```python
from build123d import *

# Parameters (mm, degrees)
SKETCH1_W                = 180
SKETCH1_H                = 110
BOSS_EXTRUDE1_DEPTH      = 50
BOSS_EXTRUDE2_DEPTH      = 110
CUT_EXTRUDE1_DEPTH       = 146.344418537
BOSS_EXTRUDE5_DEPTH      = 10
BOSS_EXTRUDE5_DEPTH_BACK = 10
SKETCH5_R                = 5
SKETCH6_W                = 218.788065493
SKETCH6_H                = 71.8794134
CUT_EXTRUDE2_DEPTH       = 126


with BuildPart() as part:
    # Sketch1 → Boss-Extrude1 (new body)
    with BuildSketch(Plane(origin=(0, 0, 0), x_dir=(1, 0, 0), z_dir=(0, 1, 0))):
        Rectangle(SKETCH1_W, SKETCH1_H)
    extrude(amount=BOSS_EXTRUDE1_DEPTH)

    # Sketch2 → Boss-Extrude2 (add)
    with BuildSketch(Plane(origin=(-35, 0, -55), x_dir=(1, 0, 0), z_dir=(0, 0, 1))):
        with BuildLine():
            Line((-55, 0), (125, 0))
            ThreePointArc((125, 0), (35, -50), (-55, 0))
        make_face()
    extrude(amount=BOSS_EXTRUDE2_DEPTH)

    # Sketch3 → Cut-Extrude1 (cut, through all)
    with BuildSketch(Plane(origin=(0, 50, 0), x_dir=(1, 0, 0), z_dir=(0, 1, 0))):
        Polygon((-49.118803686, -55), (-90, 15.808309091), (-90, -55), align=None)
    cut_extrude1 = extrude(amount=-CUT_EXTRUDE1_DEPTH, mode=Mode.SUBTRACT)

    # Mirror1: Cut-Extrude1 across plane
    add(cut_extrude1.mirror(Plane(origin=(0, 0, 0), x_dir=(0, 0, 1), z_dir=(1, 0, 0))), mode=Mode.SUBTRACT)

    # Sketch5 → Boss-Extrude5 (add, two sides: drawn at the far end of the back side and taken through both)
    with BuildSketch(Plane(origin=(0, 0, -55), x_dir=(-1, 0, 0), z_dir=(0, 0, -1)).offset(-BOSS_EXTRUDE5_DEPTH_BACK)):
        Circle(SKETCH5_R)
    extrude(amount=BOSS_EXTRUDE5_DEPTH + BOSS_EXTRUDE5_DEPTH_BACK)

    # Sketch4 → Revolve1 (revolve)
    with BuildSketch(Plane(origin=(-60.654801368, 0, 35.019065898), x_dir=(0.49999999999999495, 0, 0.8660254037844417), z_dir=(-0.8660254037844417, 0, 0.49999999999999495))):
        with BuildLine():
            ThreePointArc((-20.965161058, 42.942576489), (4.034838942, 17.942576489), (-20.965161058, -7.057423511))
            Line((-20.965161058, -7.057423511), (-20.965161058, 42.942576489))
        make_face()
    revolve1 = revolve(axis=Axis((-71.137381897, 42.942576489, 16.862703827), (0, -1, 0)))

    # Mirror2: Revolve1 across plane
    add(revolve1.mirror(Plane(origin=(0, 0, 0), x_dir=(0, 0, 1), z_dir=(1, 0, 0))))

    # Sketch6 → Cut-Extrude2 (cut)
    with BuildSketch(Plane(origin=(0, 50, 0), x_dir=(1, 0, 0), z_dir=(0, 1, 0))):
        with Locations((-0.333721882, -20.131397609)):
            Rectangle(SKETCH6_W, SKETCH6_H)
    extrude(amount=-CUT_EXTRUDE2_DEPTH, mode=Mode.SUBTRACT)


solid = part.part
```
Design review of the part built by this model. Coordinates are the model's own, in mm. A direction names the side the tool comes from. Give positions to 0.01 mm unless a question says otherwise; leave off trailing zeros. Write each loop counter-clockwise with the first axis right and the second up, starting at its lowest first coordinate (ties: lowest second). Pieces come first, ordered by that corner, then holes. Notation, with made-up numbers: (-11, 80) - (39, 80) arc R13 ccw to (39, 90) - close; hole circle Ø7 at (-5.75, 33.5). An arc over 180 degrees is marked (long way). Return JSON: item names as keys, results as strings. Group by question number.
(1) We need section A-A, the plane x = 0. Give the boundary of the cut face in (y, z), then the cut area to 3 significant figures.
(2) Insertion check: pin 1 (10 mm diameter, centred on x = 40.5, z = -21.5, fed in from -Y); pin 2 (1 mm diameter, centred on y = -19.5, z = -45.5, fed in from -X); pin 3 (4 mm diameter, centred on x = 70.5, z = -49, fed in from -Y). Each pin has a flat end and moves straight along its axis. Give the tip position at first contact, or say it passes through.
(3) To check wall thickness, follow probe 1 along Z at (x, y) = (76.5, -1); probe 2 along X at (y, z) = (-4, -60.5); probe 3 along X at (y, z) = (-38, -50). State the ranges of each line that lie inside material, in increasing order.
(4) We need section D-D, the plane x = 56. Give the boundary of the cut face in (y, z).
(5) We need section B-B, the plane y = 3. Give the boundary of the cut face in (x, z), then the cut area to 3 significant figures.
(6) We need section C-C, the plane z = -49.5. Give the boundary of the cut face in (x, y), then the cut area to 3 significant figures.
(7) Machinability: for faces 1 (the cylindrical face through (1.08, -4.88, -59.93)), 2 (the flat face through (90, 25, -35)), which of the approach directions +Z, -Z, +X, -X, +Y, -Y give a long, thin tool a straight path to every point of the face, cutting with its end or side? Answer none if there is none.
Reported:
{
 "1": {"outline": "(-50, -55) - (-5, -55) - (-5, -65) - (5, -65) - (5, -55) - (50, -55) - (50, -15.81) - (-50, -15.81) - close", "area": "4,020 mm2"},
 "2": {"pin 1": "stops at y = -43.88", "pin 2": "stops at x = -74.91", "pin 3": "stops at y = -24.89"},
 "3": {"probe 1": "z = -55 to -15.81", "probe 2": "x = -3 to 3", "probe 3": "x = -48.99 to 48.99"},
 "4": {"outline": "(-34, -55) - (50, -55) - (50, -15.81) - (-34, -15.81) - close"},
 "5": {"outline": "(-90, -55) - (-4, -55) - (-4, -65) - (4, -65) - (4, -55) - (90, -55) - (90, -15.81) - (-90, -15.81) - close", "area": "7,130 mm2"},
 "6": {"outline": "(-90, 0) arc R106 ccw to (90, 0) - (90, 50) - (-90, 50) - close", "area": "15,400 mm2"},
 "7": {"face 1": "-Z", "face 2": "+Z, -Z, +X, +Y, -Y"}
}
